from build123d import *

# Parameters (mm, degrees)
SKETCH1_W           = 125
SKETCH1_H           = 35
BOSS_EXTRUDE1_DEPTH = 4
BOSS_EXTRUDE2_DEPTH = 8
SKETCH4_R           = 6
BOSS_EXTRUDE3_DEPTH = 1
SKETCH5_R           = 3.95
BOSS_EXTRUDE4_DEPTH = 7
BOSS_EXTRUDE5_DEPTH = 27


with BuildPart() as part:
    # Sketch1 → Boss-Extrude1 (new body)
    with BuildSketch(Plane(origin=(0, 0, 0), x_dir=(1, 0, 0), z_dir=(0, 1, 0))):
        with Locations((62.5, 17.5)):
            Rectangle(SKETCH1_W, SKETCH1_H)
    extrude(amount=BOSS_EXTRUDE1_DEPTH)

    # Sketch3 → Boss-Extrude2 (add)
    with BuildSketch(Plane.XY):
        with BuildLine():
            Line((50.210098614, 36.599902553), (27.398199936, 4))
            Line((27.398199936, 4), (97.601800064, 4))
            Line((97.601800064, 4), (74.789901386, 36.599902553))
            ThreePointArc((74.789901386, 36.599902553), (62.5, 43), (50.210098614, 36.599902553))
        make_face()
    extrude(amount=-BOSS_EXTRUDE2_DEPTH)

    # Sketch4 → Boss-Extrude3 (add)
    with BuildSketch(Plane(origin=(0, 0, -8), x_dir=(-1, 0, 0), z_dir=(0, 0, -1))):
        with Locations(Location((-62.5, 28, 0), (0, 0, 180))):
            Circle(SKETCH4_R)
    extrude(amount=BOSS_EXTRUDE3_DEPTH)

    # Sketch5 → Boss-Extrude4 (add)
    with BuildSketch(Plane(origin=(0, 0, -9), x_dir=(-1, 0, 0), z_dir=(0, 0, -1))):
        with Locations((-62.5, 28)):
            Circle(SKETCH5_R)
    extrude(amount=BOSS_EXTRUDE4_DEPTH)

    # Sketch8 → Boss-Extrude5 (add)
    with BuildSketch(Plane(origin=(0, 0, -8), x_dir=(-1, 0, 0), z_dir=(0, 0, -1))):
        with BuildLine():
            Line((-51.277701451, 4), (-27.398199936, 4))
            Line((-27.398199936, 4), (-33.049223109, 12.07573308))
            Line((-33.049223109, 12.07573308), (-41.325541145, 12.07573308))
            ThreePointArc((-41.325541145, 12.07573308), (-45.805934025, 7.427004448), (-51.277701451, 4))
        make_face()
        with BuildLine():
            Line((-91.950776891, 12.07573308), (-83.674458855, 12.07573308))
            ThreePointArc((-83.674458855, 12.07573308), (-79.194065975, 7.427004448), (-73.722298549, 4))
            Line((-73.722298549, 4), (-97.601800064, 4))
            Line((-97.601800064, 4), (-91.950776891, 12.07573308))
        make_face()
    extrude(amount=BOSS_EXTRUDE5_DEPTH)


solid = part.part
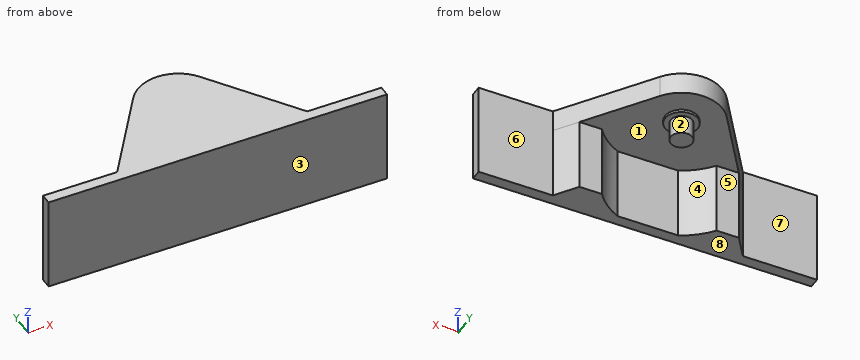
Here's how the part is built. I have some questions about the finished solid (model axes, mm). Face numbers are marked on the shaded views. A direction names the side the tool comes from. Coordinates: 2 decimals unless noted, no trailing zeros. Order: outer loops, then holes, each group sorted by start corner. A loop starts at its lowest first (then second) coordinate and runs counter-clockwise, first axis right, second up. Notation, with made-up numbers: (26, 73.5) - (80, 73.5) arc R33 ccw to (80, 108.5) - close; hole circle Ø10 at (12, 52.5). An arc over 180 degrees is marked (long way). Use CSV: the item, a comma, the result in double quotes. Start each with the question number.
1. Suppose I cut it at C-C on y = 9. List the corners of the cut face in (x, z) for me, then the cut area to 3 significant figures.
2. Suppose I cut it at B-B on x = 62.5. List the corners of the cut face in (y, z) for me.
3. Suppose I cut it at D-D on z = -27.5. List the corners of the cut face in (x, y) for me.
4. Suppose I cut it at A-A on z = -10.5. List the corners of the cut face in (x, y) for me.
5. I'm going to push flat-ended pins straight in: pin 1 (3.5 mm diameter, centred on x = 63, y = 29.5, fed in from -Z); pin 2 (2.5 mm diameter, centred on x = 35, z = -18, fed in from +Y); pin 3 (8 mm diameter, centred on x = 22.5, z = -16.5, fed in from +Y). Where does each tip first touch, or does it pass through?
6. If we mould it in two halves opening along X, with no side actions, what happens to the marked faces 1, 2, 3 and 4? For each: +X half, -X half, draft (parallel to the pull), parting line (faces both ways), or undercut.
7. For the marked faces 5, 6, 7 and 8, which set-ups out of +Z, -Z, +X, -X, +Y, -Y let a thin tool reach every point of the face, with its end or its side?
8. Please list where these lines run through material, in increasing order: line 1 (Z direction, x = 73, y = 23); line 2 (Y direction, x = 84.5, z = -15.5); line 3 (Y direction, x = 19.5, z = -2). Write a range as from..to.
Output:
1,outline,"(30.9, -35) - (44.04, -35) - (44.04, -8) - (80.96, -8) - (80.96, -35) - (94.1, -35) - (94.1, 0) - (30.9, 0) - close"
1,area,"1,220 mm2"
2,outline,"(0, -35) - (4, -35) - (4, -8) - (22, -8) - (22, -9) - (24.05, -9) - (24.05, -16) - (31.95, -16) - (31.95, -9) - (34, -9) - (34, -8) - (43, -8) - (43, 0) - (0, 0) - close"
3,outline,"(0, 0) - (125, 0) - (125, 4) - (97.6, 4) - (91.95, 12.08) - (83.67, 12.08) arc R26.49 cw to (73.72, 4) - (51.28, 4) arc R26.49 cw to (41.33, 12.08) - (33.05, 12.08) - (27.4, 4) - (0, 4) - close"
4,outline,"(0, 0) - (125, 0) - (125, 4) - (97.6, 4) - (91.95, 12.08) - (83.67, 12.08) arc R26.49 cw to (73.72, 4) - (51.28, 4) arc R26.49 cw to (41.33, 12.08) - (33.05, 12.08) - (27.4, 4) - (0, 4) - close; circle Ø7.9 at (62.5, 28)"
5,pin 1,"stops at z = -16"
5,pin 2,"stops at y = 12.08"
5,pin 3,"stops at y = 4"
6,face 1,"undercut"
6,face 2,"parting line"
6,face 3,"draft"
6,face 4,"undercut"
7,face 5,"-Z, +X, -X, +Y"
7,face 6,"+Z, -Z, +X, +Y"
7,face 7,"+Z, -Z, -X, +Y"
7,face 8,"-Z, +X, -X, +Y, -Y"
8,line 1,"z = -8..0"
8,line 2,"y = 0..12.08"
8,line 3,"y = 0..4"
